Build history of the part. All positions in model axes, mm. A direction names the side the tool comes from. Round coordinates to 2 decimals unless told otherwise and drop trailing zeros. Loops run counter-clockwise (first coordinate to the right, second up) from the corner with the lowest first, then second, coordinate; pieces in that order, holes last. Notation, with made-up numbers: (40.5, 60.5) - (60.5, 60.5) arc R24 cw to (60.5, 84.5) - close; hole circle Ø11 at (18, 52). An arc over 180 degrees is marked (long way). Put each result on its own line as item: value. Start each with the question number.
from build123d import *

# Parameters (mm, degrees)
BOSS_EXTRUDE2_DEPTH            = 140
HOLE_FOR_M5_300_SC_NUTS_SP_1_D = 5
HOLE_FOR_M5_300_SC_NUTS_SP_2_D = 5


with BuildPart() as part:
    # Sketch2 → Boss-Extrude2 (new body)
    with BuildSketch(Plane.XY):
        Polygon((-10.037935248, 20.448337429), (-10.037935248, -1.551662571), (18.962064752, -1.551662571), (18.962064752, -4.551662571), (-13.037935248, -4.551662571), (-13.037935248, 20.448337429), align=None)
    extrude(amount=BOSS_EXTRUDE2_DEPTH)

    # Hole for M5 300® SC Nuts (SP)1 (through all)
    with Locations(Plane(origin=(8.962064752, -1.551662571, 15), x_dir=(0, 0, 1), z_dir=(0, 1, 0))):
        with Locations((0, 0), (32, 0), (78, 0), (110, 0)):
            Hole(HOLE_FOR_M5_300_SC_NUTS_SP_1_D / 2)

    # Hole for M5 300® SC Nuts (SP)2 (through all)
    with Locations(Plane(origin=(-10.037935248, 0, 0), x_dir=(0, 0, -1), z_dir=(1, 0, 0))):
        with Locations((-20, 8.448337429), (-70, 8.448337429), (-120, 8.448337429)):
            Hole(HOLE_FOR_M5_300_SC_NUTS_SP_2_D / 2)


solid = part.part
Item 1: Drop flat-ended pins along their axis: pin 1 Ø4 at (x, z) = (8.96, 15) entering from +Y; pin 2 Ø1.5 at (y, z) = (14, 17.5) entering from +X; pin 3 Ø8.5 at (x, z) = (0, 99) entering from +Y. Give the stop position or say it passes through.
Item 2: Slice it at B-B (z = 37). Give the cut face in (x, y), plus the area to 3 significant figures.
Item 3: Drill centre lines: probe 1 along X at (y, z) = (-3.85, 125); probe 2 along Y at (x, z) = (-11, 70); probe 3 along X at (y, z) = (0.75, 49). Where is each one in solid material? Low to high. Write a range as [from, to].
Item 4: Which spindle directions (+Z, -Z, +X, -X, +Y, -Y) get a long thin tool onto all of the face, cutting with end or side? Do faces 4 (the flat face through (-13.038, 5, 69)), 5 (the flat face through (4, -1.552, 69)). Say none if no direction does.
Item 5: Slice it at A-A (z = 70). Give the cut face in (x, y).
Item 6: Two-plate mould, pull along X, no slides. Class faces 1 (the cylindrical face through (9.713, -3.073, 122.615)), 2 (the flat face through (18.962, -3, 69)), 3 (the flat face through (-3, -2, 140)): pulls with the +X half, pulls with the -X half, needs draft (parallel to the pull), parting line crosses it, or undercut.
Computed values:
1. pin 1: passes through
1. pin 2: stops at x = -10.04
1. pin 3: stops at y = -1.55
2. outline: (-13.04, -4.55) - (18.96, -4.55) - (18.96, -1.55) - (-10.04, -1.55) - (-10.04, 20.45) - (-13.04, 20.45) - close
2. area: 162 mm^2
3. probe 1: x = [-13.04, 6.46], [11.46, 18.96]
3. probe 2: y = [-4.55, 5.95], [10.95, 20.45]
3. probe 3: x = [-13.04, -10.04]
4. face 4: +Z, -Z, -X, +Y, -Y
4. face 5: +Z, -Z, +X, +Y
5. outline: (-13.04, -4.55) - (18.96, -4.55) - (18.96, -1.55) - (-10.04, -1.55) - (-10.04, 5.95) - (-13.04, 5.95) - close; (-13.04, 10.95) - (-10.04, 10.95) - (-10.04, 20.45) - (-13.04, 20.45) - close
6. face 1: undercut
6. face 2: pulls with the +X half
6. face 3: needs draft
